For this review, take the finished solid that the model builds, in its own axes (mm). Face numbers are marked on the shaded views. A direction names the side the tool comes from. Round coordinates to 2 decimals unless told otherwise and drop trailing zeros. Order: outer loops, then holes, each group sorted by start corner. A loop starts at its lowest first (then second) coordinate and runs counter-clockwise, first axis right, second up. Notation, with made-up numbers: M 36,19.5 L 46,19.5 A16 ccw 46,40.5 Z; hole C 81.5,35.25 d10. An arc over 180 degrees is marked long. Put each result on its own line as item: value.
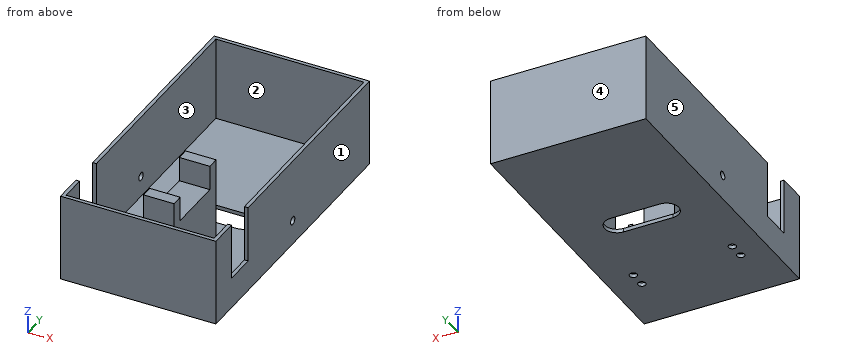
from build123d import *

# Parameters (mm, degrees)
SKETCH1_W                  = 63
SKETCH1_H                  = 118
BOSS_EXTRUDE1_DEPTH        = 35.5
SKETCH2_W                  = 60
SKETCH2_H                  = 115
CUT_EXTRUDE1_DEPTH         = 34
SKETCH3_W                  = 12.4
SKETCH3_H                  = 3.3
SKETCH3_H_2                = 1.5
SKETCH3_H_3                = 22.75
BOSS_EXTRUDE2_DEPTH        = 33.18
CUT_EXTRUDE2_REACH         = 129.081
SKETCH4_W                  = 10
SKETCH4_H                  = 22.75
CUT_EXTRUDE3_REACH         = 138.738
SKETCH5_W                  = 22.87
SKETCH5_H                  = 12.89
CUT_EXTRUDE4_REACH         = 138.738
SKETCH6_W                  = 22.87
SKETCH6_H                  = 12.89
CUT_EXTRUDE5_DEPTH         = 137.435882377
M2_5_CLEARANCE_HOLE1_D     = 3.05
M2_5_CLEARANCE_HOLE1_DEPTH = 35.5
M3_CLEARANCE_HOLE1_D       = 3.2512
M3_CLEARANCE_HOLE1_DEPTH   = 1.5
M3_CLEARANCE_HOLE2_D       = 3.2512
M3_CLEARANCE_HOLE2_DEPTH   = 63


with BuildPart() as part:
    # Sketch1 → Boss-Extrude1 (new body)
    with BuildSketch(Plane.XY.offset(34)):
        with Locations((30, 57.5)):
            Rectangle(SKETCH1_W, SKETCH1_H)
    extrude(amount=-BOSS_EXTRUDE1_DEPTH)

    # Sketch2 → Cut-Extrude1 (cut)
    with BuildSketch(Plane.XY.offset(34)):
        with Locations((30, 57.5)):
            Rectangle(SKETCH2_W, SKETCH2_H)
    extrude(amount=-CUT_EXTRUDE1_DEPTH, mode=Mode.SUBTRACT)

    # Sketch3 → Boss-Extrude2 (add)
    with BuildSketch(Plane.XY):
        with Locations((30, 15.9)):
            Rectangle(SKETCH3_W, SKETCH3_H)
        with Locations((30, 18.3)):
            Rectangle(SKETCH3_W, SKETCH3_H_2)
        with Locations((30, 30.425)):
            Rectangle(SKETCH3_W, SKETCH3_H_3)
        with Locations((30, 44.95)):
            Rectangle(SKETCH3_W, SKETCH3_H)
        with Locations((30, 42.55)):
            Rectangle(SKETCH3_W, SKETCH3_H_2)
    extrude(amount=BOSS_EXTRUDE2_DEPTH)

    # Sketch4 → Cut-Extrude2 (cut, up to next)
    with BuildSketch(Plane.ZY.offset(-23.8), mode=Mode.PRIVATE) as cut_extrude2_sk1:
        with Locations((28.18, 30.425)):
            Rectangle(SKETCH4_W, SKETCH4_H)
    cut_extrude2_tool1 = extrude(cut_extrude2_sk1.sketch, amount=-CUT_EXTRUDE2_REACH, mode=Mode.PRIVATE) & part.part
    add(cut_extrude2_tool1.solids().sort_by_distance((23.8, 30.425, 28.18))[0], mode=Mode.SUBTRACT)

    # Sketch5 → Cut-Extrude3 (cut, up to next)
    with BuildSketch(Plane(origin=(61.5, 0, 0), x_dir=(0, 0, -1), z_dir=(1, 0, 0)), mode=Mode.PRIVATE) as cut_extrude3_sk1:
        with Locations((-22.565, 16.805)):
            Rectangle(SKETCH5_W, SKETCH5_H)
    cut_extrude3_tool1 = extrude(cut_extrude3_sk1.sketch, amount=-CUT_EXTRUDE3_REACH, mode=Mode.PRIVATE) & part.part
    add(cut_extrude3_tool1.solids().sort_by_distance((61.5, 16.805, 22.565))[0], mode=Mode.SUBTRACT)

    # Sketch6 → Cut-Extrude4 (cut, up to next)
    with BuildSketch(Plane.ZY.offset(1.5), mode=Mode.PRIVATE) as cut_extrude4_sk1:
        with Locations((22.565, 16.805)):
            Rectangle(SKETCH6_W, SKETCH6_H)
    cut_extrude4_tool1 = extrude(cut_extrude4_sk1.sketch, amount=-CUT_EXTRUDE4_REACH, mode=Mode.PRIVATE) & part.part
    add(cut_extrude4_tool1.solids().sort_by_distance((-1.5, 16.805, 22.565))[0], mode=Mode.SUBTRACT)

    # Sketch7 → Cut-Extrude5 (cut, through all)
    with BuildSketch(Plane(origin=(0, 0, -1.5), x_dir=(-1, 0, 0), z_dir=(0, 0, -1))):
        with BuildLine():
            Line((-40, 55), (-20, 55))
            ThreePointArc((-20, 55), (-15, 60), (-20, 65))
            Line((-20, 65), (-40, 65))
            ThreePointArc((-40, 65), (-45, 60), (-40, 55))
        make_face()
    extrude(amount=-CUT_EXTRUDE5_DEPTH, mode=Mode.SUBTRACT)

    # M2.5 Clearance Hole1
    with Locations(Plane(origin=(0, 0, -1.5), x_dir=(-1, 0, 0), z_dir=(0, 0, -1))):
        with Locations((-9.95, 28.42), (-9.95, 21.935), (-50.05, 28.42), (-50.05, 21.935)):
            Hole(M2_5_CLEARANCE_HOLE1_D / 2, depth=M2_5_CLEARANCE_HOLE1_DEPTH)

    # M3 Clearance Hole1
    with Locations(Plane(origin=(0, 0, 0), x_dir=(0, 0, -1), z_dir=(1, 0, 0))):
        with Locations((-8.5, 57.5)):
            Hole(M3_CLEARANCE_HOLE1_D / 2, depth=M3_CLEARANCE_HOLE1_DEPTH)

    # M3 Clearance Hole2
    with Locations(Plane(origin=(61.5, 0, 0), x_dir=(0, 0, -1), z_dir=(1, 0, 0))):
        with Locations((-8.5, 57.5)):
            Hole(M3_CLEARANCE_HOLE2_D / 2, depth=M3_CLEARANCE_HOLE2_DEPTH)


solid = part.part
(1) Draft analysis for pull direction X (two halves, no side actions). For the marked faces 3, 4 and 5, state which applies: released by +X, released by -X, zero draft, split by the parting line, or undercut.
A:
face 3: undercut
face 4: zero draft
face 5: released by -X
(2) To check wall thickness, follow L1, parallel to Y at x = 33.5, z = 19.5; L2, parallel to X at y = 39, z = 16; L3, parallel to Y at x = 32.5, z = 30. State the ranges of each line that lie inside material, in increasing order.
A:
L1: y = -1.5 to 0, 14.25 to 46.6, 115 to 116.5
L2: x = -1.5 to 0, 23.8 to 36.2, 60 to 61.5
L3: y = -1.5 to 0, 14.25 to 19.05, 41.8 to 46.6, 115 to 116.5
(3) Add section B-B on z = 18. Give the boundary of the cut face in (x, y), then the cut area to 3 significant figures.
A:
outline: M -1.5,-1.5 L 61.5,-1.5 L 61.5,10.36 L 60,10.36 L 60,0 L 0,0 L 0,10.36 L -1.5,10.36 Z; M -1.5,23.25 L 0,23.25 L 0,115 L 60,115 L 60,23.25 L 61.5,23.25 L 61.5,116.5 L -1.5,116.5 Z; M 23.8,14.25 L 36.2,14.25 L 36.2,46.6 L 23.8,46.6 Z
area: 896 mm2
(4) Add section D-D on z = 31. Give the boundary of the cut face in (x, y).
A:
outline: M -1.5,-1.5 L 61.5,-1.5 L 61.5,10.36 L 60,10.36 L 60,0 L 0,0 L 0,10.36 L -1.5,10.36 Z; M -1.5,23.25 L 0,23.25 L 0,115 L 60,115 L 60,23.25 L 61.5,23.25 L 61.5,116.5 L -1.5,116.5 Z; M 23.8,14.25 L 36.2,14.25 L 36.2,19.05 L 23.8,19.05 Z; M 23.8,41.8 L 36.2,41.8 L 36.2,46.6 L 23.8,46.6 Z
(5) Insertion check: pin 1 Ø1.4 at (x, y) = (30.5, 17.5) entering from +Z; pin 2 Ø3 at (x, y) = (49, 67) entering from +Z; pin 3 Ø1.6 at (x, y) = (-1, 17) entering from +Z. Each pin has a flat end and moves straight along its axis. Give the tip position at first contact, or say it passes through.
A:
pin 1: stops at z = 33.18
pin 2: stops at z = 0
pin 3: stops at z = 11.13
(6) Add section C-C on x = 26.5. Give the boundary of the cut face in (y, z).
A:
outline: M -1.5,-1.5 L 55,-1.5 L 55,0 L 46.6,0 L 46.6,33.18 L 41.8,33.18 L 41.8,23.18 L 19.05,23.18 L 19.05,33.18 L 14.25,33.18 L 14.25,0 L 0,0 L 0,34 L -1.5,34 Z; M 65,-1.5 L 116.5,-1.5 L 116.5,34 L 115,34 L 115,0 L 65,0 Z
(7) For the marked faces 1 and 2, list the 3-axis set-ups (+Z, -Z, +X, -X, +Y, -Y) from which the entire face can be reached by the end or side of a thin tool; tool diameter is ignored.
A:
face 1: +Z, -Z, +X, +Y, -Y
face 2: +Z
(8) Add section A-A on y = 28.42. Give the boundary of the cut face in (x, z) (3 decimals), then the cut area to 3 significant figures.
A:
outline: M -1.5,-1.5 L 8.425,-1.5 L 8.425,0 L 0,0 L 0,34 L -1.5,34 Z; M 11.475,-1.5 L 48.525,-1.5 L 48.525,0 L 36.2,0 L 36.2,23.18 L 23.8,23.18 L 23.8,0 L 11.475,0 Z; M 51.575,-1.5 L 61.5,-1.5 L 61.5,34 L 60,34 L 60,0 L 51.575,0 Z
area: 475 mm2
